Source: three-view drawing plus pictorial views. Frame: mm from the lowest corner of the part. A direction names the side the tool comes from. Round coordinates to 2 decimals unless told otherwise and drop trailing zeros. Loops run counter-clockwise (first coordinate to the right, second up) from the corner with the lowest first, then second, coordinate; pieces in that order, holes last. Notation, with made-up numbers: (52, -27.5) -> (83, -27.5) arc R18 cw to (83, -17.5) -> close; hole circle Ø11 at (-29.5, 75). An arc over 180 degrees is marked (long way). One line per question, with ' | ' between items. Start each with the question number.
Q1. Cut plane D-D on y = 17. Return loops of the section in (x, z).
Q2. Cut plane A-A on x = 9.5. Return loops of the section in (y, z), and give its area (3 significant figures).
Q3. Access query for the marked faces 1 and 2. Directions: +Z, -Z, +X, -X, +Y, -Y. A direction counts if a zero-diameter tool reaches every point of the face in a straight line with its end or side. Return the directions, or none.
Q4. Material intervals for L1, parallel to Z at x = 7.25, y = 2.5; L2, parallel to X at y = 9.5, z = 10.5; L3, parallel to X at y = 7.25, z = 37.5, sorted ascending.
Q5. Cut plane C-C on z = 23. Return loops of the section in (x, y), and give its area (3 significant figures).
Q6. Contact query for flat-ended pins moving along their axis: P1, Ø2, axis at y = 10, z = 45, coming from the +X side; P2, Ø2, axis at y = 13, z = 14.5, coming from the +X side; P3, Ø6, axis at x = 9.5, z = 58, coming from the +Y side. Output: stop coordinate, or through.
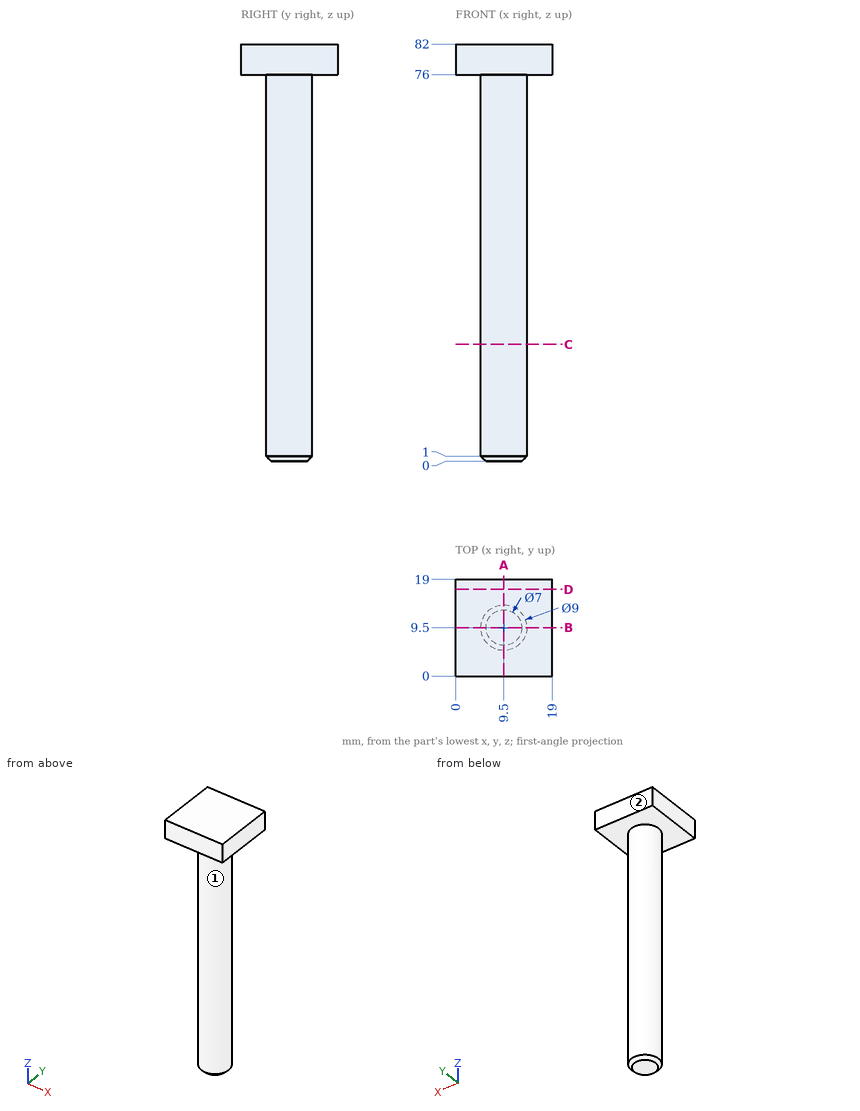
Results:
1) outline: (0, 76) -> (19, 76) -> (19, 82) -> (0, 82) -> close
2) outline: (0, 76) -> (5, 76) -> (5, 1) -> (6, 0) -> (13, 0) -> (14, 1) -> (14, 76) -> (19, 76) -> (19, 82) -> (0, 82) -> close | area: 797 mm^2
3) face 1: -Z | face 2: +Z, -Z, +X, -X, +Y
4) L1: 76 to 82 | L2: 5 to 14 | L3: 5.6 to 13.4
5) outline: circle Ø9 at (9.5, 9.5) | area: 63.6 mm^2
6) P1: x = 14 | P2: x = 13.24 | P3: y = 14
